Part model, mm, in its own coordinate system. Give positions to 0.01 mm unless a question says otherwise; leave off trailing zeros. Order: outer loops, then holes, each group sorted by start corner. A loop starts at its lowest first (then second) coordinate and runs counter-clockwise, first axis right, second up.
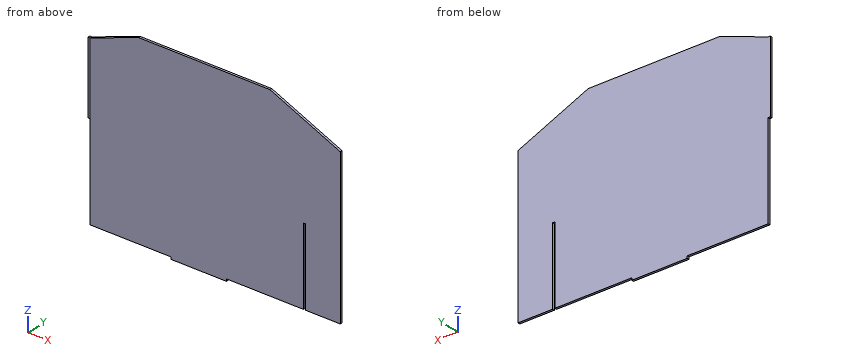
from build123d import *

# Parameters (mm, degrees)
SKETCH1_W           = 308.1112
SKETCH1_H           = 3.175
BOSS_EXTRUDE1_DEPTH = 267.83
SKETCH3_W           = 155.702
SKETCH3_H           = 3.175
BOSS_EXTRUDE3_DEPTH = 3.175
SKETCH4_W           = 50.038
SKETCH4_H           = 3.175
BOSS_EXTRUDE4_DEPTH = 267.83
CUT_EXTRUDE1_DEPTH  = 339.67870035
SKETCH8_W           = 80
SKETCH8_H           = 3.175
BOSS_EXTRUDE6_DEPTH = 3.175
CUT_EXTRUDE3_DEPTH  = 339.67870035
SKETCH13_W          = 104.779999964
SKETCH13_H          = 3.1854967
BOSS_EXTRUDE7_DEPTH = 3.175


with BuildPart() as part:
    # Sketch1 → Boss-Extrude1 (new body)
    with BuildSketch(Plane.XY):
        Rectangle(SKETCH1_W, SKETCH1_H)
    extrude(amount=BOSS_EXTRUDE1_DEPTH)

    # Sketch3 → Boss-Extrude3 (add)
    with BuildSketch(Plane(origin=(154.0556, 0, 0), x_dir=(0, 0, -1), z_dir=(1, 0, 0))):
        with Locations((-189.979, 0)):
            Rectangle(SKETCH3_W, SKETCH3_H)
    extrude(amount=BOSS_EXTRUDE3_DEPTH)

    # Sketch4 → Boss-Extrude4 (add)
    with BuildSketch(Plane.XY.offset(267.83)):
        with Locations((182.2496, 0)):
            Rectangle(SKETCH4_W, SKETCH4_H)
    extrude(amount=-BOSS_EXTRUDE4_DEPTH)

    # Sketch6 → Cut-Extrude1 (cut, through all)
    with BuildSketch(Plane(origin=(0, 1.5875, 0), x_dir=(1, 0, 0), z_dir=(0, 1, 0))):
        Polygon((207.2686, -223.38), (105.6686, -267.83), (207.2686, -267.83), align=None)
    extrude(amount=-CUT_EXTRUDE1_DEPTH, mode=Mode.SUBTRACT)

    # Sketch8 → Boss-Extrude6 (add)
    with BuildSketch(Plane(origin=(0, 0, 0), x_dir=(-1, 0, 0), z_dir=(0, 0, -1))):
        with Locations((-2.78399998, 0)):
            Rectangle(SKETCH8_W, SKETCH8_H)
    extrude(amount=BOSS_EXTRUDE6_DEPTH)

    # Sketch11 → Cut-Extrude3 (cut, through all)
    with BuildSketch(Plane.XZ.offset(1.5875)):
        Polygon((-154.0556, 242.43), (-84.2056, 267.83), (-154.0556, 267.83), align=None)
    extrude(amount=-CUT_EXTRUDE3_DEPTH, mode=Mode.SUBTRACT)

    # Sketch13 → Boss-Extrude7 (add)
    with BuildSketch(Plane.ZY.offset(154.0556)):
        with Locations((190.040000018, -0.00524835)):
            Rectangle(SKETCH13_W, SKETCH13_H)
    extrude(amount=BOSS_EXTRUDE7_DEPTH)


solid = part.part
Item 1: Drill centre lines: probe 1 along X at (y, z) = (-0.6, 107.5); probe 2 along Y at (x, z) = (80.5, 214); probe 3 along Z at (x, y) = (72, 0.75). Where is each one in solid material? Low to high.
Item 2: Band-saw the part on C-C on x = 174.5. List the corners of the cut face in (y, z), plus the area to 3 significant figures.
Item 3: Band-saw the part on B-B on y = -0.55. List the corners of the cut face in (x, z) (3 decimals), plus the area to 3 significant figures.
Item 4: Band-saw the part on A-A on z = 50. List the corners of the cut face in (x, y).
Item 5: Drop flat-ended pins along their axis: P1, Ø1.6, axis at x = 155.5, y = 1, coming from the -Z side; P2, Ø4, axis at x = -45.5, z = 53, coming from the -Y side; P3, Ø1, axis at x = 189, y = 0, coming from the -Z side. Give the stop position or say it passes through.
Item 6: Band-saw the part on D-D on x = -101.5. List the corners of the cut face in (y, z), plus the area to 3 significant figures.
Working result:
1. probe 1: x = -154.06 to 154.06, 157.23 to 207.27
1. probe 2: y = -1.59 to 1.59
1. probe 3: z = 0 to 267.83
2. outline: (-1.59, 0) - (1.59, 0) - (1.59, 237.72) - (-1.59, 237.72) - close
2. area: 755 mm2
3. outline: (-157.231, 137.65) - (-154.056, 137.65) - (-154.056, 0) - (-37.216, 0) - (-37.216, -3.175) - (42.784, -3.175) - (42.784, 0) - (154.056, 0) - (154.056, 112.128) - (157.231, 112.128) - (157.231, 0) - (207.269, 0) - (207.269, 223.38) - (105.669, 267.83) - (-84.206, 267.83) - (-154.056, 242.43) - (-157.231, 242.43) - close
3. area: 93,900 mm2
4. outline: (-154.06, -1.59) - (154.06, -1.59) - (154.06, 1.59) - (-154.06, 1.59) - close; (157.23, -1.59) - (207.27, -1.59) - (207.27, 1.59) - (157.23, 1.59) - close
5. P1: stops at z = 112.13
5. P2: stops at y = -1.59
5. P3: stops at z = 0
6. outline: (-1.59, 0) - (1.59, 0) - (1.59, 261.54) - (-1.59, 261.54) - close
6. area: 830 mm2
